from build123d import *

# Parameters (mm, degrees)
F0_R      = 10
F0_R_2    = 6.55
F1_DEPTH  = 30
F0_R_3    = 2.6
F2_DEPTH  = 26
F3_W      = 7
F3_H      = 30
F3_W_2    = 30
F4_DEPTH  = 7
F5_DEPTH  = 30
F6_W      = 40
F6_H      = 5
F7_DEPTH  = 23
F9_DEPTH  = 25
F10_R     = 3.15
F11_DEPTH = 25
F12_R     = 3.15
F13_DEPTH = 25
F15_DEPTH = 30.001


with BuildPart() as f1:
    # F0 (on Top) → F1 (new body)
    with BuildSketch(Plane.XY):
        Circle(F0_R)
        Circle(F0_R_2, mode=Mode.SUBTRACT)
    extrude(amount=F1_DEPTH)

    # F0 (on Top) → F2 (join)
    with BuildSketch(Plane.XY):
        Circle(F0_R_2)
        Circle(F0_R_3, mode=Mode.SUBTRACT)
    extrude(amount=F2_DEPTH)

    # F3 (on Top) → F4 (join)
    with BuildSketch(Plane.XY):
        with BuildLine():
            Line((11.4, -15), (11.4, 15))
            Line((11.4, 15), (0, 10))
            ThreePointArc((0, 10), (7.071068, 7.071068), (10, 0))
            ThreePointArc((10, 0), (7.071068, -7.071068), (0, -10))
            Line((0, -10), (11.4, -15))
        make_face()
        with Locations((14.9, 0)):
            Rectangle(F3_W, F3_H)
        with Locations((33.4, 0)):
            Rectangle(F3_W_2, F3_H)
    extrude(amount=F4_DEPTH)

    # F3 (on Top) → F5 (join)
    with BuildSketch(Plane.XY):
        with Locations((14.9, 0)):
            Rectangle(F3_W, F3_H)
    extrude(amount=-F5_DEPTH)

    # F6 (on face) → F7 (join, through all)
    with BuildSketch(Plane.XY.offset(7)):
        with Locations((28.4, 0)):
            Rectangle(F6_W, F6_H)
    extrude(amount=F7_DEPTH)

    # F8 (on face) → F9 (cut)
    with BuildSketch(Plane.XZ.offset(2.5)):
        Polygon((48.4, 30), (9.682458, 30), (48.4, 7), align=None)
    extrude(amount=-F9_DEPTH, mode=Mode.SUBTRACT)

    # F10 (on face) → F11 (cut)
    with BuildSketch(Plane.YZ.offset(18.4)):
        with Locations((-7.5, -15)):
            Circle(F10_R)
        with Locations((7.5, -15)):
            Circle(F10_R)
    extrude(amount=-F11_DEPTH, mode=Mode.SUBTRACT)

    # F12 (on face) → F13 (cut)
    with BuildSketch(Plane.XY):
        with Locations((33.4, -7.5)):
            Circle(F12_R)
        with Locations((33.4, 7.5)):
            Circle(F12_R)
    extrude(amount=F13_DEPTH, mode=Mode.SUBTRACT)

    # F14 (on face) → F15 (cut, through all)
    with BuildSketch(Plane.XZ.offset(15)):
        Polygon((51.2021, -41.370519), (48.4, 0), (-16.937578, 0), (-15.380099, -41.370519), align=None)
    extrude(amount=-F15_DEPTH, mode=Mode.SUBTRACT)


solid = f1.part
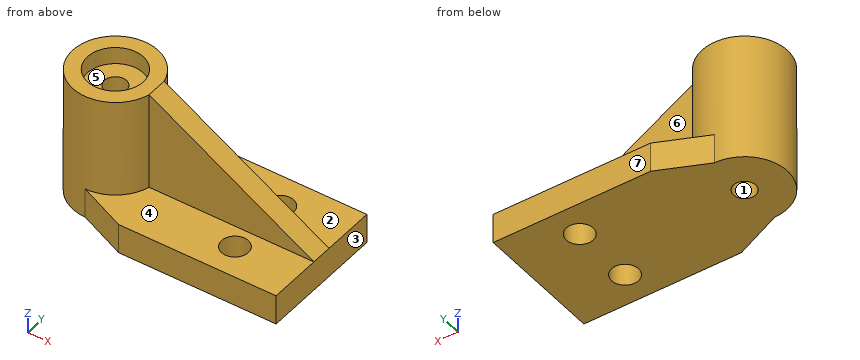
Read the model definition and answer for the solid it produces. Units are mm, in the model's axes. Face numbers are marked on the shaded views. A direction names the side the tool comes from. Coordinates: 2 decimals unless noted, no trailing zeros. Order: outer loops, then holes, each group sorted by start corner. A loop starts at its lowest first (then second) coordinate and runs counter-clockwise, first axis right, second up. Notation, with made-up numbers: (25.25, 16.5) -> (80.25, 16.5) arc R15 ccw to (80.25, 23.5) -> close; hole circle Ø3 at (-33, -10). An arc over 180 degrees is marked (long way). Answer as a JSON object with one key per item and string values.
1) A cutting plane is placed at D-D, the plane x = 19. Determine the outline of the cut face in (y, z), plus the area to 3 significant figures.
Model answer:
{"outline": "(-15, 0) -> (15, 0) -> (15, 7) -> (2.5, 7) -> (2.5, 24.46) -> (-2.5, 24.46) -> (-2.5, 7) -> (-15, 7) -> close", "area": "297 mm²"}
2) Each of these flat-tipped pins is pushed along its axis until it touches: pin 1 (4 mm diameter, centred on x = 0, y = 2, fed in from +Z); pin 2 (1 mm diameter, centred on x = 16, y = -8.5, fed in from +Z); pin 3 (8 mm diameter, centred on y = 11, z = 18.5, fed in from -X); pin 4 (4 mm diameter, centred on x = 33.4, y = -7.5, fed in from -Z). Where does it stop, or does it pass through?
Model answer:
{"pin 1": "stops at z = 26", "pin 2": "stops at z = 7", "pin 3": "stops at x = -7.14", "pin 4": "passes through"}
3) The mould has two halves that part along X. Classify the marked faces 1, 2 and 3: released by +X, released by -X, zero draft, split by the parting line, or undercut.
Model answer:
{"face 1": "undercut", "face 2": "zero draft", "face 3": "released by +X"}
4) A cutting plane is placed at C-C, the plane y = -1.75. Determine the outline of the cut face in (x, z), plus the area to 3 significant figures.
Model answer:
{"outline": "(-9.85, 0) -> (-1.92, 0) -> (-1.92, 26) -> (-6.31, 26) -> (-6.31, 30) -> (-9.85, 30) -> close; (1.92, 0) -> (48.4, 0) -> (48.4, 7) -> (9.68, 30) -> (6.31, 30) -> (6.31, 26) -> (1.92, 26) -> close", "area": "1,150 mm²"}
5) A cutting plane is placed at A-A, the plane z = 3.75. Determine the outline of the cut face in (x, y).
Model answer:
{"outline": "(0, -10) -> (11.4, -15) -> (48.4, -15) -> (48.4, 15) -> (11.4, 15) -> (0, 10) arc R10 ccw to start; hole circle Ø5.2 at (0, 0); hole circle Ø6.3 at (33.4, -7.5); hole circle Ø6.3 at (33.4, 7.5)"}
6) A cutting plane is placed at B-B, the plane x = 34.5. Determine the outline of the cut face in (y, z), plus the area to 3 significant figures.
Model answer:
{"outline": "(-15, 0) -> (-10.45, 0) -> (-10.45, 7) -> (-15, 7) -> close; (-4.55, 0) -> (4.55, 0) -> (4.55, 7) -> (2.5, 7) -> (2.5, 15.26) -> (-2.5, 15.26) -> (-2.5, 7) -> (-4.55, 7) -> close; (10.45, 0) -> (15, 0) -> (15, 7) -> (10.45, 7) -> close", "area": "169 mm²"}
7) A tool of negligible diameter and unlimited length cuts with its end or side. For the marked faces 4, 5, 6 and 7, from which of +Z, -Z, +X, -X, +Y, -Y can it reach the whole face along a straight path? Write none if from no direction.
Model answer:
{"face 4": "+Z, +X, -Y", "face 5": "+Z", "face 6": "+Z, +X, +Y", "face 7": "+Z, -Z, +X, -X, +Y"}
8) Consider line 1 along Y through (x, z) = (0, 18); line 2 along Y through (x, z) = (0, 27.35); line 3 along Z through (x, y) = (40, 8.5). Determine where each line is inside the solid, lowest interval first. Write a range as from..to.
Model answer:
{"line 1": "y = -10..-2.6, 2.6..10", "line 2": "y = -10..-6.55, 6.55..10", "line 3": "z = 0..7"}
